Part print with two shaded views. Sizes in mm from the minimum x, y, z corner. Round coordinates to 2 decimals unless told otherwise and drop trailing zeros. Write each loop counter-clockwise with the first axis right and the second up, starting at its lowest first coordinate (ties: lowest second). Pieces come first, ordered by that corner, then holes. Notation, with made-up numbers: (78, 69) -> (85, 69) arc R14 ccw to (85, 82) -> close; hole circle Ø2 at (-0.75, -1). An arc over 180 degrees is marked (long way). Answer in a Markdown table with one row per item.
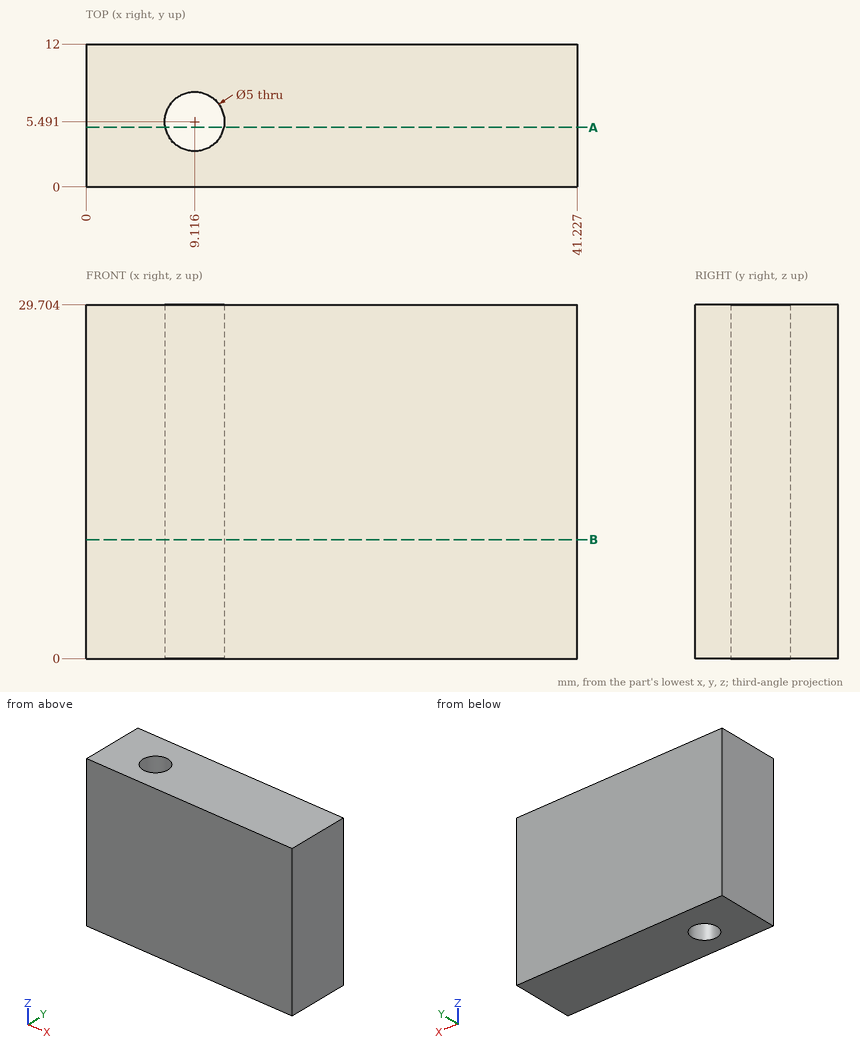
Q1. Wall check: line 1 (Y direction, x = 9, z = 7); line 2 (X direction, y = 4.75, z = 15.25); line 3 (X direction, y = 7.25, z = 11.75) (1 decimal). Give the ranges that are in metal, low to high. Write a range as [from, to].
A:
| item | result |
|---|---|
| line 1 | [0, 2.99], [7.99, 12] |
| line 2 | [0, 6.73], [11.5, 41.23] |
| line 3 | [0, 7.3], [10.9, 41.2] |
Q2. Saw through at B-B on z = 10. Write the cut outline in (x, y) (1 decimal), plus the area to 3 significant figures.
A:
| item | result |
|---|---|
| outline | (0, 0) -> (41.2, 0) -> (41.2, 12) -> (0, 12) -> close; hole circle Ø5 at (9.1, 5.5) |
| area | 475 mm² |
Q3. Saw through at A-A on y = 5. Write the cut outline in (x, z) (1 decimal), plus the area to 3 significant figures.
A:
| item | result |
|---|---|
| outline | (0, 0) -> (6.7, 0) -> (6.7, 29.7) -> (0, 29.7) -> close; (11.6, 0) -> (41.2, 0) -> (41.2, 29.7) -> (11.6, 29.7) -> close |
| area | 1,080 mm² |
